The model under review builds one solid part; all positions refer to its coordinate system, in mm. A direction names the side the tool comes from. Coordinates: 2 decimals unless noted, no trailing zeros. Order: outer loops, then holes, each group sorted by start corner. A loop starts at its lowest first (then second) coordinate and runs counter-clockwise, first axis right, second up. Notation, with made-up numbers: M -2.5,38.5 L 6.5,38.5 A30 ccw 6.5,70.5 Z; hole C 78,-35 d6. An arc over 180 degrees is marked long. One line per item, written item: value.
```python
from build123d import *

# Parameters (mm, degrees)
SKETCH_W         = 33
SKETCH_H         = 20
PAD_DEPTH        = 14
FILLET_R         = 8
FILLET001_R      = 8
FILLET002_R      = 8
FILLET003_R      = 8
POCKET_DEPTH     = 5.51
SKETCH002_R      = 4
POCKET001_DEPTH  = 8.491
SKETCH003_R      = 2
POCKET002_DEPTH  = 14.001
CHAMFER_SIZE2    = 3
CHAMFER_SIZE     = 2
CHAMFER001_SIZE2 = 3
CHAMFER001_SIZE  = 2
FILLET004_R      = 0.5
SKETCH004_R      = 6.5
POCKET003_DEPTH  = 0.01


with BuildPart() as part:
    # Sketch → Pad (new body)
    with BuildSketch(Plane.XY):
        Rectangle(SKETCH_W, SKETCH_H)
    extrude(amount=PAD_DEPTH)

    # Fillet
    fillet_edges = [part.edges().sort_by_distance(p)[0] for p in [
        (-16.5, -10, 7),
    ]]
    fillet(fillet_edges, radius=FILLET_R)

    # Fillet001
    fillet001_edges = [part.edges().sort_by_distance(p)[0] for p in [
        (16.5, -10, 7),
    ]]
    fillet(fillet001_edges, radius=FILLET001_R)

    # Fillet002
    fillet002_edges = [part.edges().sort_by_distance(p)[0] for p in [
        (16.5, 10, 7),
    ]]
    fillet(fillet002_edges, radius=FILLET002_R)

    # Fillet003
    fillet003_edges = [part.edges().sort_by_distance(p)[0] for p in [
        (-16.5, 10, 7),
    ]]
    fillet(fillet003_edges, radius=FILLET003_R)

    # Sketch001 (on Face10 of Fillet003) → Pocket (cut)
    with BuildSketch(Plane.XY.offset(14)):
        Polygon((-6.5, 3.752777), (-6.5, -3.752777), (0, -7.505553), (6.5, -3.752777), (6.5, 3.752777), (0, 7.505553), align=None)
    extrude(amount=-POCKET_DEPTH, mode=Mode.SUBTRACT)

    # Sketch002 (on Face17 of Pocket) → Pocket001 (cut, through all)
    with BuildSketch(Plane.XY.offset(8.49)):
        Circle(SKETCH002_R)
    extrude(amount=-POCKET001_DEPTH, mode=Mode.SUBTRACT)

    # Sketch003 (on Face11 of Pocket001) → Pocket002 (cut, through all)
    with BuildSketch(Plane.XY.offset(14)):
        with Locations((-11.5, 0)):
            Circle(SKETCH003_R)
        with Locations((11.5, 0)):
            Circle(SKETCH003_R)
    extrude(amount=-POCKET002_DEPTH, mode=Mode.SUBTRACT)

    # Chamfer
    chamfer_edges = [part.edges().sort_by_distance(p)[0] for p in [
        (9.5, 0, 0),
    ]]
    chamfer_side = part.faces().sort_by_distance((0, 9.614124, 0))[0]
    chamfer(chamfer_edges, length=CHAMFER_SIZE, length2=CHAMFER_SIZE2, reference=chamfer_side)

    # Chamfer001
    chamfer001_edges = [part.edges().sort_by_distance(p)[0] for p in [
        (-13.5, 0, 0),
    ]]
    chamfer001_side = part.faces().sort_by_distance((7.114124, 0, 0))[0]
    chamfer(chamfer001_edges, length=CHAMFER001_SIZE, length2=CHAMFER001_SIZE2, reference=chamfer001_side)

    # Fillet004
    fillet004_edges = [part.edges().sort_by_distance(p)[0] for p in [
        (0, 10, 0),
        (-16.5, 0, 0),
        (0, -10, 0),
        (16.5, 0, 0),
    ]]
    fillet(fillet004_edges, radius=FILLET004_R)

    # Sketch004 (on Face24 of Fillet004) → Pocket003 (cut)
    with BuildSketch(Plane.XY.offset(14)):
        Circle(SKETCH004_R)
    extrude(amount=-POCKET003_DEPTH, mode=Mode.SUBTRACT)


solid = part.part
```
(1) For L1, parallel to X at y = -2, z = 2; L2, parallel to Y at x = 0, z = 2; L3, parallel to X at y = 2.25, z = 13, list the stretches that pass through material, from the lowest coordinate up.
Geometry results:
L1: x = -16.5 to -13.26, -9.74 to -3.46, 3.46 to 9.74, 13.26 to 16.5
L2: y = -10 to -4, 4 to 10
L3: x = -16.5 to -6.5, 6.5 to 16.5
(2) Mouldability with a two-part tool opening along Y and no side actions: class faces 1 (the cylindrical face through (14.219, 7.594, 7.344)), 2 (the flat face through (-3.2, 5.66, 11.28)), 3 (the flat face through (7, 0, 14)), 4 (the flat face through (6.5, 0, 11)) as +Y half, -Y half, draft (parallel to the pull), parting line (faces both ways), or undercut.
Geometry results:
face 1: +Y half
face 2: undercut
face 3: draft
face 4: undercut
(3) We need section D-D, the plane y = 1.25. Count the separate pieces of the cut face and the enclosed holes in it, plus the area to 3 significant figures.
Geometry results:
separate pieces: 4
enclosed holes: 0
area: 224 mm2
(4) Insertion check: pin 1 Ø8 at (x, z) = (13, 5.5) entering from -Y; pin 2 Ø9 at (x, y) = (0, 0) entering from +Z; pin 3 Ø10 at (x, y) = (11.5, 1.5) entering from +Z; pin 4 Ø1 at (y, z) = (-5, 2) entering from -X. Each pin has a flat end and moves straight along its axis. Give the tip position at first contact, or say it passes through.
Geometry results:
pin 1: stops at y = -9.98
pin 2: stops at z = 8.49
pin 3: stops at z = 14
pin 4: stops at x = -16.1
(5) We need section B-B, the plane x = -1. State the section outline as (y, z) points.
Geometry results:
outline: M -10,0.5 A0.5 ccw -9.5,0 L -3.87,0 L -3.87,8.49 L -6.93,8.49 L -6.93,14 L -10,14 Z; M 3.87,0 L 9.5,0 A0.5 ccw 10,0.5 L 10,14 L 6.93,14 L 6.93,8.49 L 3.87,8.49 Z
(6) We need section C-C, the plane z = 9.25. State the section outline as (x, y) points.
Geometry results:
outline: M -16.5,-2 A8 ccw -8.5,-10 L 8.5,-10 A8 ccw 16.5,-2 L 16.5,2 A8 ccw 8.5,10 L -8.5,10 A8 ccw -16.5,2 Z; hole C -11.5,0 d4; hole M -6.5,-3.75 L 0,-7.51 L 6.5,-3.75 L 6.5,3.75 L 0,7.51 L -6.5,3.75 Z; hole C 11.5,0 d4
(7) Tool access review of faces 5 (the flat face through (-3.3, -5.6, 11.3)), 6 (the flat face through (-16.5, 0, 7)): name each direction out of +Z, -Z, +X, -X, +Y, -Y from which nothing blocks a thin tool from reaching the whole face with its end or side.
Geometry results:
face 5: +Z
face 6: +Z, -Z, -X, +Y, -Y
(8) We need section A-A, the plane z = 4.75. State the section outline as (x, y) points, plus the area to 3 significant figures.
Geometry results:
outline: M -16.5,-2 A8 ccw -8.5,-10 L 8.5,-10 A8 ccw 16.5,-2 L 16.5,2 A8 ccw 8.5,10 L -8.5,10 A8 ccw -16.5,2 Z; hole C -11.5,0 d4; hole C 0,0 d8; hole C 11.5,0 d4
area: 530 mm2
